Geometry check sheet. Reference: the model listing, model coordinates, mm. Face numbers are marked on the shaded views. Round coordinates to 2 decimals unless told otherwise and drop trailing zeros. Write each loop counter-clockwise with the first axis right and the second up, starting at its lowest first coordinate (ties: lowest second). Pieces come first, ordered by that corner, then holes. Notation, with made-up numbers: (4, 48) -> (57, 48) arc R20 ccw to (57, 60) -> close; hole circle Ø3 at (41.5, 79.5). An arc over 180 degrees is marked (long way). Return JSON: item names as keys, results as strings. Group by question number.
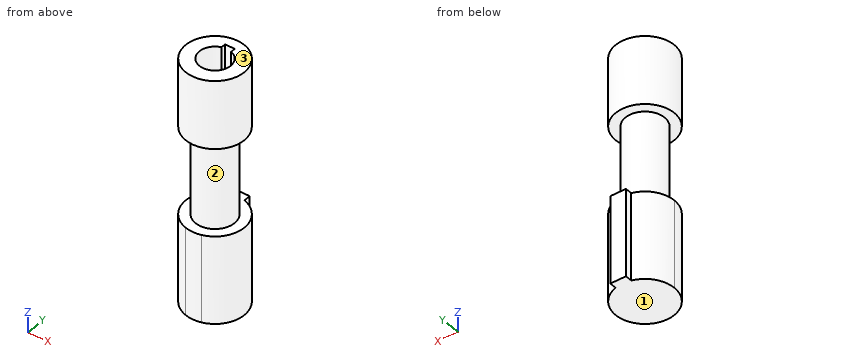
from build123d import *

# Parameters (mm, degrees)
SKETCH1_R                = 15
BOSS_EXTRUDE1_DEPTH      = 35
BOSS_EXTRUDE3_DEPTH      = 1
SKETCH2_R                = 10
BOSS_EXTRUDE4_DEPTH      = 50
BOSS_EXTRUDE5_DEPTH      = 40
BOSS_EXTRUDE5_DEPTH_BACK = 5
SKETCH4_R                = 10
CUT_EXTRUDE2_DEPTH       = 30


with BuildPart() as part:
    # Sketch1 → Boss-Extrude1 (new body)
    with BuildSketch(Plane.XY):
        Circle(SKETCH1_R)
        with BuildLine():
            Line((-2.5, 10), (2.5, 10))
            Line((2.5, 10), (2.5, 7.599342077))
            ThreePointArc((2.5, 7.599342077), (6.480740698, 4.69041576), (8, 0))
            ThreePointArc((8, 0), (-4.69041576, -6.480740698), (-2.5, 7.599342077))
            Line((-2.5, 7.599342077), (-2.5, 10))
        make_face(mode=Mode.SUBTRACT)
    extrude(amount=BOSS_EXTRUDE1_DEPTH)

    # Sketch1_6 → Boss-Extrude3 (add)
    with BuildSketch(Plane.XY):
        with BuildLine():
            Line((2.5, 7.599342077), (2.5, 10))
            Line((2.5, 10), (-2.5, 10))
            Line((-2.5, 10), (-2.5, 7.599342077))
            ThreePointArc((-2.5, 7.599342077), (0, 8), (2.5, 7.599342077))
        make_face()
    extrude(amount=BOSS_EXTRUDE3_DEPTH)

    # Sketch2 → Boss-Extrude4 (add)
    with BuildSketch(Plane.XY):
        Circle(SKETCH2_R)
    extrude(amount=-BOSS_EXTRUDE4_DEPTH)

    # Sketch3 → Boss-Extrude5 (add, two sides: drawn at the far end of the back side and taken through both)
    with BuildSketch(Plane(origin=(0, 0, -50), x_dir=(-1, 0, 0), z_dir=(0, 0, -1)).offset(-BOSS_EXTRUDE5_DEPTH_BACK)):
        with BuildLine():
            ThreePointArc((15, 0), (11.937336386, 9.082951062), (4, 14.456832295))
            Line((4, 14.456832295), (4, -14.456832295))
            ThreePointArc((4, -14.456832295), (11.937336386, -9.082951062), (15, 0))
        make_face()
        with BuildLine():
            Line((-4, -14.456832295), (-4, 14.456832295))
            ThreePointArc((-4, 14.456832295), (-15, 0), (-4, -14.456832295))
        make_face()
        with BuildLine():
            ThreePointArc((4, 14.456832295), (0, 15), (-4, 14.456832295))
            Line((-4, 14.456832295), (-4, -14.456832295))
            ThreePointArc((-4, -14.456832295), (0, -15), (4, -14.456832295))
            Line((4, -14.456832295), (4, 14.456832295))
        make_face()
        with BuildLine():
            Line((4, 18), (-4, 18))
            Line((-4, 18), (-4, 14.456832295))
            ThreePointArc((-4, 14.456832295), (0, 15), (4, 14.456832295))
            Line((4, 14.456832295), (4, 18))
        make_face()
    extrude(amount=BOSS_EXTRUDE5_DEPTH + BOSS_EXTRUDE5_DEPTH_BACK)

    # Sketch4 → Cut-Extrude2 (cut)
    with BuildSketch(Plane(origin=(0, 0, -50), x_dir=(-1, 0, 0), z_dir=(0, 0, -1))):
        with Locations(Location((0, 0, 0), (0, 0, 180))):
            Circle(SKETCH4_R)
    extrude(amount=CUT_EXTRUDE2_DEPTH, mode=Mode.SUBTRACT)


solid = part.part
1) Go/stop test with flat-tipped pins: P1, Ø1, axis at x = -0.5, z = -30, coming from the -Y side; P2, Ø1.8, axis at y = 17, z = -68.5, coming from the -X side; P3, Ø1, axis at x = 4, y = 1, coming from the +Z side. Record where each tip stops, or that it passes through.
2) Mould release check, pull along Z, two halves, no side actions. Record for the marked faces 1, 2 and 3: +Z half, -Z half, draft (parallel to the pull), parting line (faces both ways), or undercut.
3) Sectioned sample at C-C on y = -11.5. Enter the section's corners in (x, z).
4) Sectioned sample at B-B on z = -74.5. Enter the section's corners in (x, y).
5) Sectioned sample at A-A on x = 0. Enter the section's corners in (y, z).
6) Material ranges on probe 1 along Z at (x, y) = (2, -4.5); probe 2 along Z at (x, y) = (12.75, -5); probe 3 along Y at (x, z) = (0, 13), recorded low to high. Write a range as [from, to].
Evaluation:
{
 "1": {"P1": "stops at y = -10", "P2": "stops at x = -4", "P3": "stops at z = 0"},
 "2": {"face 1": "-Z half", "face 2": "undercut", "face 3": "+Z half"},
 "3": {"outline": "(-9.63, -90) -> (9.63, -90) -> (9.63, -45) -> (-9.63, -45) -> close; (-9.63, 0) -> (9.63, 0) -> (9.63, 35) -> (-9.63, 35) -> close"},
 "4": {"outline": "(-4, 14.46) arc R15 ccw (long way) to (4, 14.46) -> (4, 18) -> (-4, 18) -> close; hole circle Ø20 at (0, 0)"},
 "5": {"outline": "(-15, -90) -> (18, -90) -> (18, -45) -> (10, -45) -> (10, 0) -> (15, 0) -> (15, 35) -> (10, 35) -> (10, 1) -> (8, 1) -> (8, 0) -> (-8, 0) -> (-8, 35) -> (-15, 35) -> (-15, 0) -> (-10, 0) -> (-10, -45) -> (-15, -45) -> close; hole (-10, -80) -> (10, -80) -> (10, -50) -> (-10, -50) -> close"},
 "6": {"probe 1": "z = [-90, -80], [-50, 0]", "probe 2": "z = [-90, -45], [0, 35]", "probe 3": "y = [-15, -8], [10, 15]"}
}
